Drawing for the job (mm, zero at the part's lowest x, y, z). Round coordinates to 2 decimals unless told otherwise and drop trailing zeros. Order: outer loops, then holes, each group sorted by start corner. A loop starts at its lowest first (then second) coordinate and runs counter-clockwise, first axis right, second up. Notation, with made-up numbers: M 21.5,54 L 54.5,54 A37 ccw 54.5,92 Z; hole C 54.25,66.25 d3. An arc over 180 degrees is marked long. Answer as CSV lines item,"result". Start each with the question number.
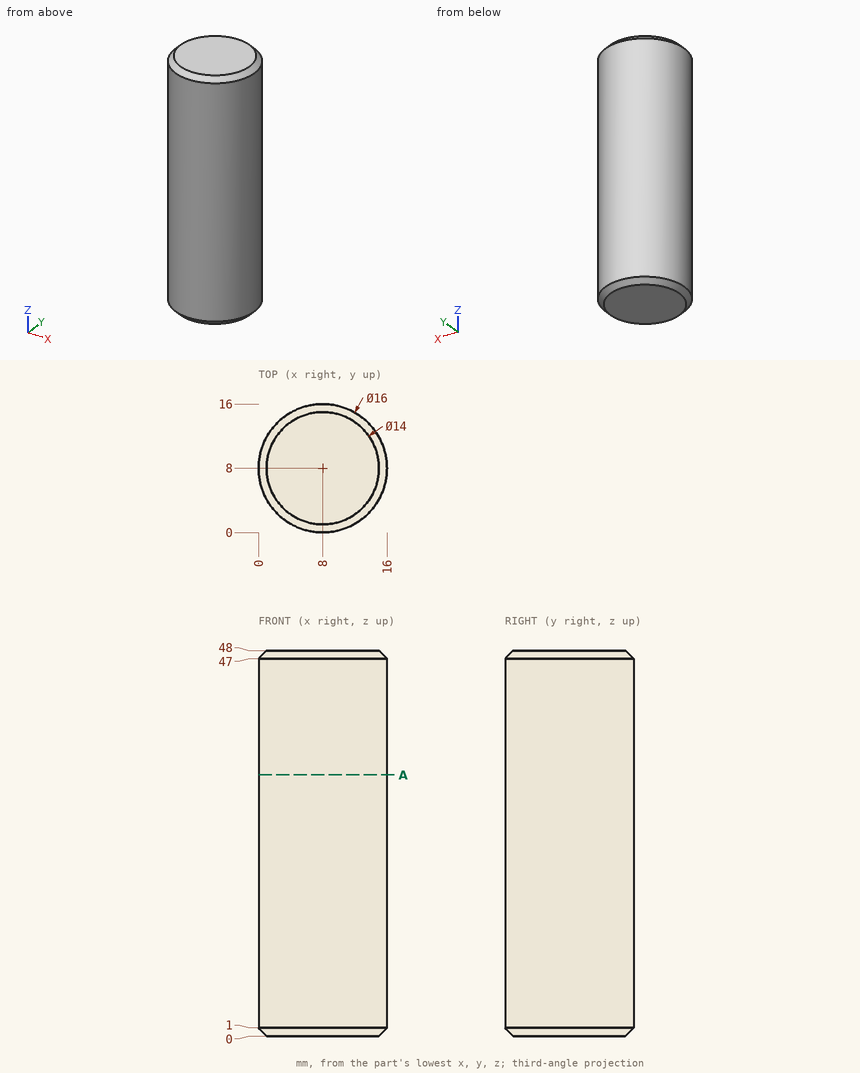
Q1. Drop flat-ended pins along their axis: P1, Ø2, axis at y = 6, z = 41, coming from the +X side; P2, Ø8, axis at y = 2, z = 37, coming from the -X side; P3, Ø1, axis at y = 12.5, z = 42, coming from the -X side. Give the stop position or say it passes through.
Q2. Band-saw the part on A-A, the plane z = 32.5. Write the cut outline in (x, y), then the cut area to 3 significant figures.
Q3. Probe line 1 along X through (y, z) = (13.5, 25); line 2 along X through (y, z) = (4.5, 2); line 3 along Y through (x, z) = (8.75, 9.5). List the from-to ranges inside material, lowest first. Write a range as from..to.
Answer:
1,P1,"stops at x = 15.94"
1,P2,"stops at x = 0.25"
1,P3,"stops at x = 1.07"
2,outline,"C 8,8 d16"
2,area,"201 mm^2"
3,line 1,"x = 2.19..13.81"
3,line 2,"x = 0.81..15.19"
3,line 3,"y = 0.04..15.96"
